from build123d import *

# Parameters (mm, degrees)
BOSS_EXTRUDE1_DEPTH = 3
SKETCH2_R           = 1.85
CUT_EXTRUDE1_DEPTH  = 71.774289117


with BuildPart() as part:
    # Sketch1 → Boss-Extrude1 (new body)
    with BuildSketch(Plane.XY):
        Polygon((14, 50), (4, 50), (4, 47), (3, 47), (3, 42), (0, 42), (0, 37), (3, 37), (3, 32), (0, 32), (0, 27), (3, 27), (3, 22), (0, 22), (0, 17), (3, 17), (3, 12), (0, 12), (0, 7), (3, 7), (3, 2), (0, 2), (0, 0), (50, 0), (50, 2), (47, 2), (47, 7), (50, 7), (50, 12), (47, 12), (47, 17), (50, 17), (50, 22), (47, 22), (47, 27), (50, 27), (50, 32), (47, 32), (47, 37), (50, 37), (50, 42), (47, 42), (47, 47), (46, 47), (46, 50), (36, 50), (36, 47), (28, 47), (28, 50), (22, 50), (22, 47), (14, 47), align=None)
    extrude(amount=BOSS_EXTRUDE1_DEPTH)

    # Sketch2 → Cut-Extrude1 (cut, through all)
    with BuildSketch(Plane.XY):
        with Locations((9, 41)):
            Circle(SKETCH2_R)
        with Locations((41, 41)):
            Circle(SKETCH2_R)
        with Locations((41, 9)):
            Circle(SKETCH2_R)
        with Locations((9, 9)):
            Circle(SKETCH2_R)
        Polygon((33.074995027, 5.5), (15.474995027, 5.5), (5.5, 16.925004973), (5.5, 34.525004973), (16.925004973, 44.5), (34.525004973, 44.5), (44.5, 33.074995027), (44.5, 15.474995027), align=None)
    extrude(amount=CUT_EXTRUDE1_DEPTH, mode=Mode.SUBTRACT)


solid = part.part
Geometry check sheet. Reference: the model listing, model coordinates, mm. A direction names the side the tool comes from. Round coordinates to 2 decimals unless told otherwise and drop trailing zeros. Order: outer loops, then holes, each group sorted by start corner. A loop starts at its lowest first (then second) coordinate and runs counter-clockwise, first axis right, second up. Notation, with made-up numbers: M 68.25,14.25 L 120.25,14.25 A11 cw 120.25,20.25 Z; hole C 41.25,55 d4. An arc over 180 degrees is marked long. Answer in a Markdown table with one row per item. Add a question column.
Item 1: Sectioned sample at D-D, the plane x = 13. Enter the section's corners in (y, z).
Item 2: Material ranges on L1, parallel to X at y = 48.5, z = 0.35; L2, parallel to Y at x = 2.5, z = 2.4; L3, parallel to X at y = 40.5, z = 0.75, recorded low to high. Write a range as [from, to].
Item 3: Sectioned sample at C-C, the plane y = 41. Enter the section's corners in (x, z).
Item 4: Draft check along X on faces 1 (the face through (50, 9, 1)), 2 (the face through (49, 2, 1)), 3 (the face through (38.87, 10.56, 1.48)). Enter one of: released by +X, released by -X, zero draft, split by the parting line, or undercut.
Item 5: Set-up check for faces 4 (the face through (26, 44.5, 1)), 5 (the face through (1, 37, 1)), 6 (the face through (47, 4, 1)), 7 (the face through (47, 44, 1)), 8 (the face through (18, 47, 1)): record each of +Z, -Z, +X, -X, +Y, -Y from which the full face is reachable in a straight line by a thin tool's end or side.
Item 6: Depth check by flat-ended pin: pin 1 Ø0.9 at (y, z) = (3.5, 1) entering from +X; pin 2 Ø1.5 at (y, z) = (49, 1) entering from -X; pin 3 Ø1 at (x, z) = (32, 1) entering from +Y. Enter the tip coordinate at first touch or a pass-through.
Item 7: Sectioned sample at A-A, the plane y = 30.5. Enter the section's corners in (x, z).
Item 8: Sectioned sample at B-B, the plane x = 41. Enter the section's corners in (y, z).
Filled in:
| question | item | result |
|---|---|---|
| 1 | outline | M 0,0 L 8.33,0 L 8.33,3 L 0,3 Z; M 41.07,0 L 50,0 L 50,3 L 41.07,3 Z |
| 2 | L1 | x = [4, 14], [22, 28], [36, 46] |
| 2 | L2 | y = [0, 2], [7, 12], [17, 22], [27, 32], [37, 42] |
| 2 | L3 | x = [0, 7.22], [10.78, 12.34], [38.02, 39.22], [42.78, 50] |
| 3 | outline | M 0,0 L 7.15,0 L 7.15,3 L 0,3 Z; M 10.85,0 L 12.92,0 L 12.92,3 L 10.85,3 Z; M 37.58,0 L 39.15,0 L 39.15,3 L 37.58,3 Z; M 42.85,0 L 50,0 L 50,3 L 42.85,3 Z |
| 4 | face 1 | released by +X |
| 4 | face 2 | zero draft |
| 4 | face 3 | undercut |
| 5 | face 4 | +Z, -Z |
| 5 | face 5 | +Z, -Z, -X |
| 5 | face 6 | +Z, -Z, +X |
| 5 | face 7 | +Z, -Z, +X, +Y |
| 5 | face 8 | +Z, -Z, +Y |
| 6 | pin 1 | stops at x = 47 |
| 6 | pin 2 | stops at x = 4 |
| 6 | pin 3 | stops at y = 47 |
| 7 | outline | M 0,0 L 5.5,0 L 5.5,3 L 0,3 Z; M 44.5,0 L 50,0 L 50,3 L 44.5,3 Z |
| 8 | outline | M 0,0 L 7.15,0 L 7.15,3 L 0,3 Z; M 10.85,0 L 12.42,0 L 12.42,3 L 10.85,3 Z; M 37.08,0 L 39.15,0 L 39.15,3 L 37.08,3 Z; M 42.85,0 L 50,0 L 50,3 L 42.85,3 Z |
